```python
from build123d import *

# Parameters (mm, degrees)
F0_R     = 12.7
F1_DEPTH = 160.02
F2_R     = 12.7
F2_R_2   = 6.35
F3_DEPTH = 134.62
F4_R     = 6.35
F4_R_2   = 2.286
F5_DEPTH = 66.04


with BuildPart() as f1:
    # F0 (on Right) → F1 (new body)
    with BuildSketch(Plane.YZ):
        Circle(F0_R)
    extrude(amount=-F1_DEPTH)

    # F2 (on face) → F3 (cut)
    with BuildSketch(Plane.YZ):
        Circle(F2_R)
        Circle(F2_R_2, mode=Mode.SUBTRACT)
    extrude(amount=-F3_DEPTH, mode=Mode.SUBTRACT)

    # F4 (on face) → F5 (cut)
    with BuildSketch(Plane.YZ):
        Circle(F4_R)
        Circle(F4_R_2, mode=Mode.SUBTRACT)
    extrude(amount=-F5_DEPTH, mode=Mode.SUBTRACT)


solid = f1.part
```
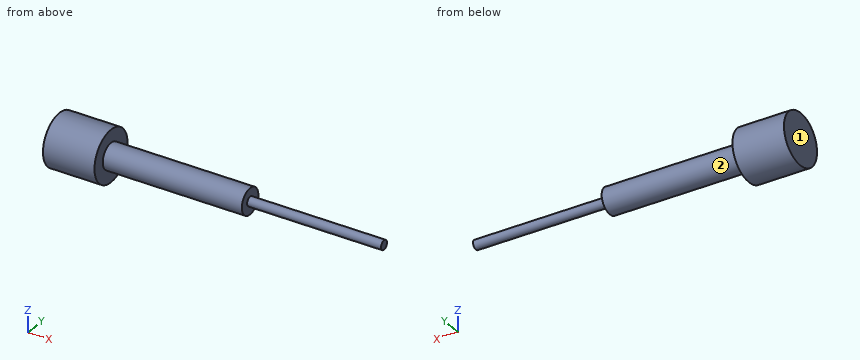
Geometry check sheet. Reference: the model listing, model coordinates, mm. Face numbers are marked on the shaded views. A direction names the side the tool comes from. Round coordinates to 2 decimals unless told otherwise and drop trailing zeros. Loops run counter-clockwise (first coordinate to the right, second up) from the corner with the lowest first, then second, coordinate; pieces in that order, holes last. Notation, with made-up numbers: (-18, -31.5) - (21, -31.5) arc R29 ccw to (21, -7.5) - close; hole circle Ø4 at (70, 63.5). An arc over 180 degrees is marked (long way). Use a Markdown table: item, result.
Q1. Access from +Z, -Z, +X, -X, +Y, -Y to the whole of each face (thin tool, end or side, straight path). Record for the marked faces 1 and 2.
Solutions:
| item | result |
|---|---|
| face 1 | +Z, -Z, -X, +Y, -Y |
| face 2 | +X |
Q2. Cross-section at B-B on x = -71. Record the cut outline in (y, z).
Solutions:
| item | result |
|---|---|
| outline | circle Ø12.7 at (0, 0) |
Q3. Cross-section at C-C on y = 8.75. Record the cut outline in (x, z).
Solutions:
| item | result |
|---|---|
| outline | (-160.02, -9.2) - (-134.62, -9.2) - (-134.62, 9.2) - (-160.02, 9.2) - close |
Q4. Cross-section at D-D on x = -42.5. Record the cut outline in (y, z).
Solutions:
| item | result |
|---|---|
| outline | circle Ø4.57 at (0, 0) |
Q5. Material ranges on line 1 (X direction, y = -10.25, z = -1.25); line 2 (X direction, y = 0.5, z = -3); line 3 (Y direction, x = -143.5, z = 11), recorded low to high.
Solutions:
| item | result |
|---|---|
| line 1 | x = -160.02 to -134.62 |
| line 2 | x = -160.02 to -66.04 |
| line 3 | y = -6.35 to 6.35 |
Q6. Go/stop test with flat-tipped pins: P1, Ø2, axis at x = -97.5, y = 9, coming from the -Z side; P2, Ø12, axis at y = -4.5, z = 3.5, coming from the +X side; P3, Ø4, axis at x = -82, y = -7, coming from the +Z side; P4, Ø5, axis at x = -97, z = 0.5, coming from the +Y side. Record where each tip stops, or that it passes through.
Solutions:
| item | result |
|---|---|
| P1 | passes through |
| P2 | stops at x = 0 |
| P3 | stops at z = 3.91 |
| P4 | stops at y = 6.35 |
Q7. Cross-section at A-A on z = 0. Record the cut outline in (x, y), plus the area to 3 significant figures.
Solutions:
| item | result |
|---|---|
| outline | (-160.02, -12.7) - (-134.62, -12.7) - (-134.62, -6.35) - (-66.04, -6.35) - (-66.04, -2.29) - (0, -2.29) - (0, 2.29) - (-66.04, 2.29) - (-66.04, 6.35) - (-134.62, 6.35) - (-134.62, 12.7) - (-160.02, 12.7) - close |
| area | 1,820 mm2 |
